Here's how the part is built. I have some questions about the finished solid (model axes, mm). Face numbers are marked on the shaded views. A direction names the side the tool comes from. Coordinates: 2 decimals unless noted, no trailing zeros. Write each loop counter-clockwise with the first axis right and the second up, starting at its lowest first coordinate (ties: lowest second). Pieces come first, ordered by that corner, then holes. Notation, with made-up numbers: M -7.5,48.5 L 3.5,48.5 A13 ccw 3.5,60.5 Z; hole C 71,64 d5. An arc over 180 degrees is marked long. Use a Markdown table: item, result.
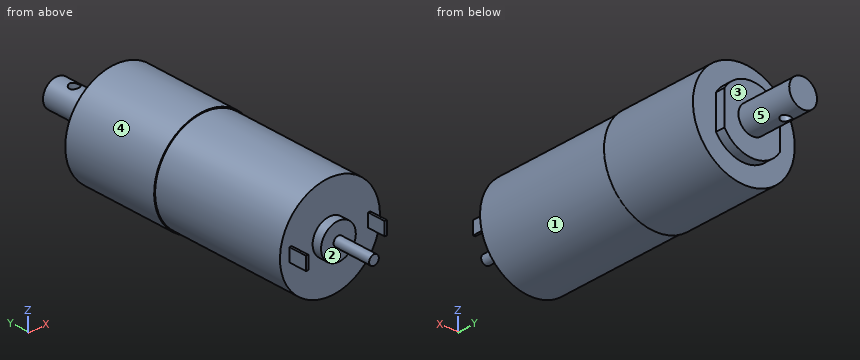
```python
from build123d import *

# Parameters (mm, degrees)
SKETCH2_R           = 10.8
BOSS_EXTRUDE1_DEPTH = 29.5
SKETCH3_R           = 11
BOSS_EXTRUDE2_DEPTH = 21
BOSS_EXTRUDE3_DEPTH = 2
SKETCH5_R           = 3
BOSS_EXTRUDE4_DEPTH = 12
SKETCH6_R           = 3.75
BOSS_EXTRUDE5_DEPTH = 2
SKETCH7_W           = 0.5
SKETCH7_H           = 2.8
BOSS_EXTRUDE6_DEPTH = 3.9
SKETCH8_R           = 1.05
BOSS_EXTRUDE7_DEPTH = 8.4
SKETCH_1_R          = 1.0375
CUT_EXTRUDE_1_DEPTH = 5


with BuildPart() as part:
    # Sketch2 → Boss-Extrude1 (new body)
    with BuildSketch(Plane(origin=(0, 0, 0), x_dir=(1, 0, 0), z_dir=(0, 1, 0))):
        with Locations(Location((0, 0, 0), (0, 0, 270))):
            Circle(SKETCH2_R)
    extrude(amount=BOSS_EXTRUDE1_DEPTH)

    # Sketch3 → Boss-Extrude2 (add)
    with BuildSketch(Plane(origin=(0, 29.5, 0), x_dir=(1, 0, 0), z_dir=(0, 1, 0))):
        with Locations(Location((0, 0, 0), (0, 0, 90))):
            Circle(SKETCH3_R)
    extrude(amount=BOSS_EXTRUDE2_DEPTH)

    # Sketch4 → Boss-Extrude3 (add)
    with BuildSketch(Plane(origin=(0, 50.5, 0), x_dir=(1, 0, 0), z_dir=(0, 1, 0))):
        with BuildLine():
            Line((6, 3.605551275), (6, -3.605551275))
            ThreePointArc((6, -3.605551275), (0, -7), (-6, -3.605551275))
            Line((-6, -3.605551275), (-6, 3.605551275))
            ThreePointArc((-6, 3.605551275), (0, 7), (6, 3.605551275))
        make_face()
    extrude(amount=BOSS_EXTRUDE3_DEPTH)

    # Sketch5 → Boss-Extrude4 (add)
    with BuildSketch(Plane(origin=(0, 52.5, 0), x_dir=(1, 0, 0), z_dir=(0, 1, 0))):
        with Locations(Location((0, 0, 0), (0, 0, 270))):
            Circle(SKETCH5_R)
    extrude(amount=BOSS_EXTRUDE4_DEPTH)

    # Sketch6 → Boss-Extrude5 (add)
    with BuildSketch(Plane.XZ):
        with Locations(Location((0, 0, 0), (0, 0, 270))):
            Circle(SKETCH6_R)
    extrude(amount=BOSS_EXTRUDE5_DEPTH)

    # Sketch7 → Boss-Extrude6 (add)
    with BuildSketch(Plane.XZ):
        with Locations((-8.5, 0)):
            Rectangle(SKETCH7_W, SKETCH7_H)
        with Locations((8.5, 0)):
            Rectangle(SKETCH7_W, SKETCH7_H)
    extrude(amount=BOSS_EXTRUDE6_DEPTH)

    # Sketch8 → Boss-Extrude7 (add)
    with BuildSketch(Plane.XZ.offset(2)):
        with Locations(Location((0, 0, 0), (0, 0, 270))):
            Circle(SKETCH8_R)
    extrude(amount=BOSS_EXTRUDE7_DEPTH)

    # 草图1 → 切除-拉伸1 (cut, symmetric)
    with BuildSketch(Plane.XY):
        with Locations(Location((0, 60.4, 0), (0, 0, 89.999999986))):
            Circle(SKETCH_1_R)
    extrude(amount=CUT_EXTRUDE_1_DEPTH, both=True, mode=Mode.SUBTRACT)


solid = part.part
```
1. Suppose I cut it at A-A on x = 0. Write out the boundary of the cut face in (y, z).
Answers follow:
| item | result |
|---|---|
| outline | M -10.4,-1.05 L -2,-1.05 L -2,-3.75 L 0,-3.75 L 0,-10.8 L 29.5,-10.8 L 29.5,-11 L 50.5,-11 L 50.5,-7 L 52.5,-7 L 52.5,-3 L 59.36,-3 L 59.36,3 L 52.5,3 L 52.5,7 L 50.5,7 L 50.5,11 L 29.5,11 L 29.5,10.8 L 0,10.8 L 0,3.75 L -2,3.75 L -2,1.05 L -10.4,1.05 Z; M 61.44,-3 L 64.5,-3 L 64.5,3 L 61.44,3 Z |
2. Suppose I cut it at C-C on z = 8. Write out the boundary of the cut face in (x, y), and give its area (3 significant figures).
Answers follow:
| item | result |
|---|---|
| outline | M -7.55,29.5 L -7.26,29.5 L -7.26,0 L 7.26,0 L 7.26,29.5 L 7.55,29.5 L 7.55,50.5 L -7.55,50.5 Z |
| area | 745 mm2 |
3. I need wall thicknesses on probe 1 along Y at (x, z) = (0.75, 5.25); probe 2 along Y at (x, z) = (-4.25, 5.75); probe 3 along X at (y, z) = (60.4, -1.5). Which ranges of each line are inside material? Lowest first, please.
Answers follow:
| item | result |
|---|---|
| probe 1 | y = 0 to 52.5 |
| probe 2 | y = 0 to 50.5 |
| probe 3 | x = -2.6 to -1.04, 1.04 to 2.6 |
4. Which directions (+Z, -Z, +X, -X, +Y, -Y) give clear straight access to the entire face, cutting with the end or side of a thin tool? Please do the marked faces 4 and 5.
Answers follow:
| item | result |
|---|---|
| face 4 | +Y, -Y |
| face 5 | +Y |
5. Will these pins go through, and if not, where does the flat tip stop? pin 1 Ø11 at (x, z) = (5, -1) entering from -Y; pin 2 Ø10 at (x, y) = (-4, 25) entering from -Z; pin 3 Ø5 at (x, z) = (-7.5, 2) entering from -Y; pin 4 Ø1 at (x, y) = (-2, 3) entering from +Z.
Answers follow:
| item | result |
|---|---|
| pin 1 | stops at y = -10.4 |
| pin 2 | stops at z = -10.85 |
| pin 3 | stops at y = -3.9 |
| pin 4 | stops at z = 10.7 |
6. We'd pull the mould along X, two halves only. Please class the marked faces 1, 2 and 3: +X half, -X half, draft (parallel to the pull), parting line (faces both ways), or undercut.
Answers follow:
| item | result |
|---|---|
| face 1 | parting line |
| face 2 | undercut |
| face 3 | draft |
7. Suppose I cut it at D-D on x = -5. Write out the boundary of the cut face in (y, z).
Answers follow:
| item | result |
|---|---|
| outline | M 0,-9.57 L 29.5,-9.57 L 29.5,-9.8 L 50.5,-9.8 L 50.5,-4.9 L 52.5,-4.9 L 52.5,4.9 L 50.5,4.9 L 50.5,9.8 L 29.5,9.8 L 29.5,9.57 L 0,9.57 Z |
